Print and shaded views of the part. All mm, measured from the part's lowest x, y and z. A direction names the side the tool comes from. Coordinates: 2 decimals unless noted, no trailing zeros. Loops run counter-clockwise (first coordinate to the right, second up) from the corner with the lowest first, then second, coordinate; pieces in that order, holes last. Notation, with made-up numbers: (14.25, 19.25) -> (29.25, 19.25) arc R20 ccw to (29.25, 25.25) -> close; hole circle Ø5 at (-19, 34). An arc over 180 degrees is marked (long way). One line per item, written item: value. Start each with the question number.
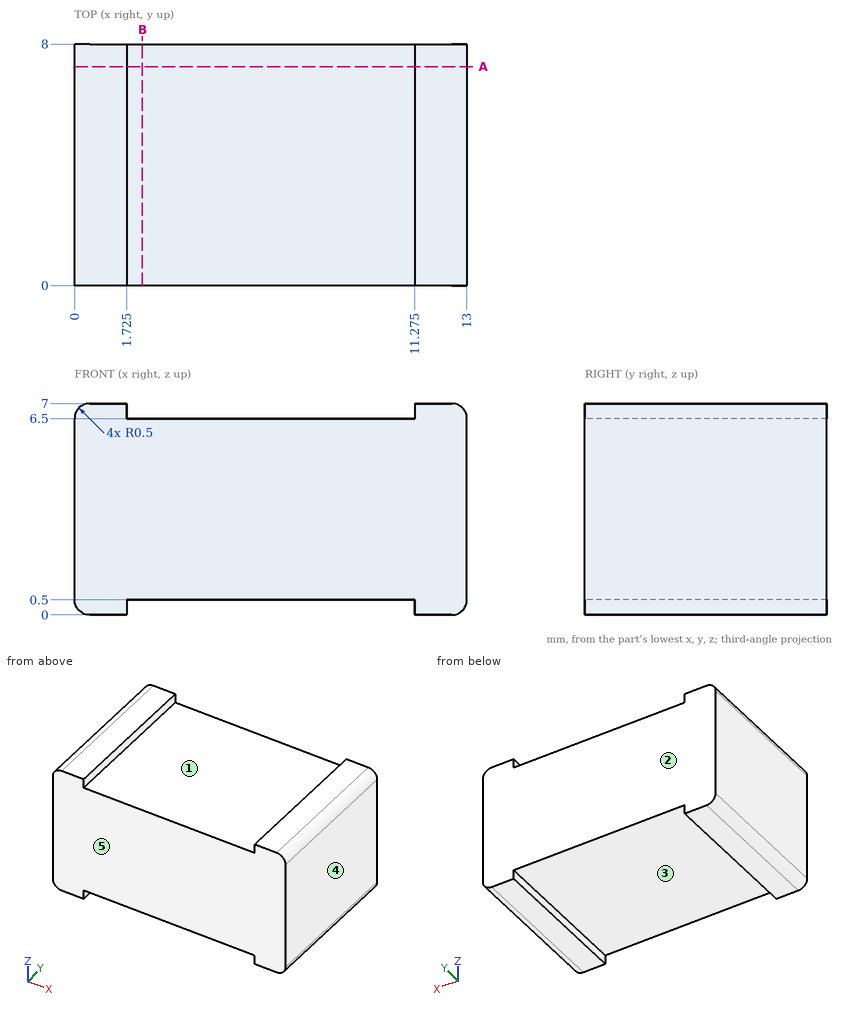
1) Pull direction X, two halves, no side cores. Call the marked faces 3, 4 and 5: +X half, -X half, draft (parallel to the pull), parting line (faces both ways), or undercut.
2) Tool access for the marked faces 1 and 2: list every direction of +Z, -Z, +X, -X, +Y, -Y with a clear straight run to the whole face (end or side of a thin tool).
3) Probe line 1 (Z direction, x = 9, y = 1.25). List the from-to ranges inside material, lowest first. Write a range as from..to.
4) Slice it at A-A (y = 7.25). Give the cut face in (x, z) (3 decimals), then the cut area to 3 significant figures.
5) Slice it at B-B (x = 2.25). Give the cut face in (y, z).
Check sheet entries:
1. face 3: undercut
1. face 4: +X half
1. face 5: draft
2. face 1: +Z, +Y, -Y
2. face 2: +Z, -Z, +X, -X, +Y
3. line 1: z = 0.5..6.5
4. outline: (0, 0.5) arc R0.5 ccw to (0.5, 0) -> (1.725, 0) -> (1.725, 0.5) -> (11.275, 0.5) -> (11.275, 0) -> (12.5, 0) arc R0.5 ccw to (13, 0.5) -> (13, 6.5) arc R0.5 ccw to (12.5, 7) -> (11.275, 7) -> (11.275, 6.5) -> (1.725, 6.5) -> (1.725, 7) -> (0.5, 7) arc R0.5 ccw to (0, 6.5) -> close
4. area: 81.2 mm^2
5. outline: (0, 0.5) -> (8, 0.5) -> (8, 6.5) -> (0, 6.5) -> close
